Source: CAD feature listing. Evaluate the final solid. Frame: model axes, mm. Give positions to 0.01 mm unless a question says otherwise; leave off trailing zeros. Answer as a JSON object with one key per item and string values. Group by question number.
1. Section query A-A (y = 189.5). Count the separate pieces of the cut face and the enclosed holes in it, plus the area to 3 significant figures.
2. Material intervals for L1, parallel to X at y = 397, z = -7; L2, parallel to Z at x = -6.5, y = 95, sorted ascending. Write a range as [from, to].
3. Pin query (flat end, axial travel): P1, Ø10, axis at x = 4.5, z = -2.5, coming from the +Y side; P2, Ø3, axis at x = -7, z = 7, coming from the +Y side; P3, Ø1, axis at x = 1.5, y = 639, coming from the -Z side. Return the tip coordinate at first contact, or that it passes through.
from build123d import *

# Parameters (mm, degrees)
SKETCH_2_W               = 20
SKETCH_2_H               = 20
EXTRUDE_20201000_DEPTH   = 1000
CUT_EXTRUDE_1005_DEPTH   = 1001.099995
PATTERN_CIRCULAR_1_COUNT = 4
SKETCH_4_R               = 2.15
CUT_EXTRUDE_4_DEPTH      = 1000


with BuildPart() as part:
    # 스케치2 → 20201000 (new body)
    with BuildSketch(Plane(origin=(0, 0, 0), x_dir=(1, 0, 0), z_dir=(0, 1, 0))):
        Rectangle(SKETCH_2_W, SKETCH_2_H)
    extrude(amount=EXTRUDE_20201000_DEPTH)

    # 스케치1 → Cut-Extrude 1005 (cut, symmetric)
    with BuildSketch(Plane(origin=(0, 0, 0), x_dir=(1, 0, 0), z_dir=(0, 1, 0))):
        with BuildLine():
            Line((4.15, 7), (-4.15, 7))
            Line((-4.15, 7), (-4.15, 4.740009506))
            ThreePointArc((-4.15, 4.740009506), (0, 3.3), (4.15, 4.740009506))
            Line((4.15, 4.740009506), (4.15, 7))
        make_face()
        Polygon((2.65, 10), (-2.65, 10), (-2.65, 8.5), (-4.15, 8.5), (-4.15, 7), (4.15, 7), (4.15, 8.5), (2.65, 8.5), align=None)
    cut_extrude_1005 = extrude(amount=CUT_EXTRUDE_1005_DEPTH, both=True, mode=Mode.SUBTRACT)

    # 원형 패턴1: Cut-Extrude 1005 ×4 about axis
    pattern_circular_1_axis = Axis((0, 0, 0), (0, 1, 0))
    for i in range(1, PATTERN_CIRCULAR_1_COUNT):
        add(cut_extrude_1005.rotate(pattern_circular_1_axis, i * 360 / PATTERN_CIRCULAR_1_COUNT), mode=Mode.SUBTRACT)

    # 스케치4 → 컷-돌출4 (cut)
    with BuildSketch(Plane.XZ):
        with BuildLine():
            ThreePointArc((9, 7), (7, 9), (5, 7))
            Line((5, 7), (7, 7))
            Line((7, 7), (7, 5))
            ThreePointArc((7, 5), (8.414213562, 5.585786438), (9, 7))
        make_face()
        with BuildLine():
            Line((7, 7), (5, 7))
            ThreePointArc((5, 7), (5.585786438, 5.585786438), (7, 5))
            Line((7, 5), (7, 7))
        make_face()
        with Locations(Location((0, 0, 0), (0, 0, 270))):
            Circle(SKETCH_4_R)
        with BuildLine():
            ThreePointArc((9, -7), (8.414213562, -5.585786438), (7, -5))
            Line((7, -5), (7, -7))
            Line((7, -7), (5, -7))
            ThreePointArc((5, -7), (7, -9), (9, -7))
        make_face()
        with BuildLine():
            Line((7, -7), (7, -5))
            ThreePointArc((7, -5), (5.585786438, -5.585786438), (5, -7))
            Line((5, -7), (7, -7))
        make_face()
        with BuildLine():
            ThreePointArc((-5, -7), (-5.585786438, -5.585786438), (-7, -5))
            Line((-7, -5), (-7, -7))
            Line((-7, -7), (-5, -7))
        make_face()
        with BuildLine():
            Line((-7, -7), (-7, -5))
            ThreePointArc((-7, -5), (-8.414213562, -8.414213562), (-5, -7))
            Line((-5, -7), (-7, -7))
        make_face()
        with BuildLine():
            Line((-7, 5), (-7, 7))
            Line((-7, 7), (-5, 7))
            ThreePointArc((-5, 7), (-8.414213562, 8.414213562), (-7, 5))
        make_face()
        with BuildLine():
            Line((-5, 7), (-7, 7))
            Line((-7, 7), (-7, 5))
            ThreePointArc((-7, 5), (-5.585786438, 5.585786438), (-5, 7))
        make_face()
    extrude(amount=-CUT_EXTRUDE_4_DEPTH, mode=Mode.SUBTRACT)


solid = part.part
Answer sheet:
{
 "1": {"separate pieces": "1", "enclosed holes": "5", "area": "146 mm^2"},
 "2": {"L1": "[-10, -9], [-5, -4.15], [4.15, 5], [9, 10]", "L2": "[-10, -8.94], [-5.06, -4.15], [4.15, 5.06], [8.94, 10]"},
 "3": {"P1": "y = 1000", "P2": "through", "P3": "z = -3.61"}
}
